Could you check a few things on this drawing? It's one solid part, dimensions in mm from its lowest x, y, z. A direction names the side the tool comes from. Coordinates: 2 decimals unless noted, no trailing zeros. Write each loop counter-clockwise with the first axis right and the second up, starting at its lowest first coordinate (ties: lowest second). Pieces come first, ordered by that corner, then holes. Notation, with made-up numbers: (69, 82.25) - (90, 82.25) arc R29 cw to (90, 119.25) - close; hole circle Ø6 at (-36.5, 69). An arc over 180 degrees is marked (long way). Answer as a JSON object with one key per item and string values. Group by question number.
1) On a 3-axis mill with a long thin cutter (end or side, diameter ignored), from which of +Z, -Z, +X, -X, +Y, -Y can I reach the whole of each face in a straight line? I mean the marked faces 1, 2 and 3. Say none if no direction works.
2) If we section it at B-B (z = 24.5): Write out the boundary of the cut face in (x, y) (1 decimal), plus the area to 3 significant figures.
3) Will these pins go through, and if not, where does the flat tip stop? pin 1 Ø1 at (y, z) = (16, 169) entering from +X; pin 2 Ø1.5 at (y, z) = (13.5, 65) entering from -X; pin 3 Ø1.2 at (y, z) = (2, 23.5) entering from +X.
4) If we section it at C-C (x = 253): Write out the boundary of the cut face in (y, z), plus the area to 3 significant figures.
5) Please list where these lines run through material, in increasing order: line 1 along Z through (x, y) = (272, 17.5); line 2 along Y through (x, z) = (126.5, 80); line 3 along Z through (x, y) = (118, 14.75) (1 decimal).
6) If we section it at D-D (z = 106.5): Write out the boundary of the cut face in (x, y), plus the area to 3 significant figures.
7) If we section it at A-A (y = 23): Write out the boundary of the cut face in (x, z) (1 decimal), plus the area to 3 significant figures.
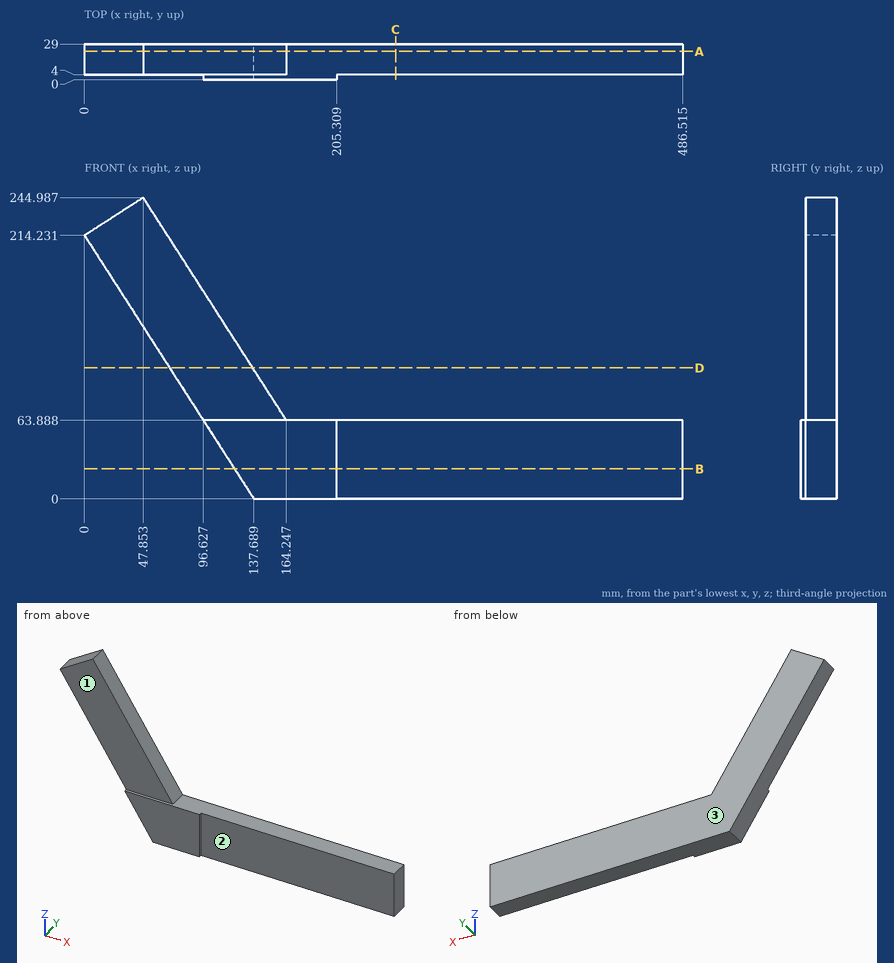
Here are the results:
{
 "1": {"face 1": "+Z, +X, -X, -Y", "face 2": "+Z, -Z, +X, -Y", "face 3": "+Z, -Z, +X, -X, +Y"},
 "2": {"outline": "(121.9, 0) - (205.3, 0) - (205.3, 4) - (486.5, 4) - (486.5, 29) - (121.9, 29) - close", "area": "9,450 mm²"},
 "3": {"pin 1": "stops at x = 97.01", "pin 2": "stops at x = 95.43", "pin 3": "stops at x = 205.31"},
 "4": {"outline": "(4, 0) - (29, 0) - (29, 63.89) - (4, 63.89) - close", "area": "1,600 mm²"},
 "5": {"line 1": "z = 0 to 63.89", "line 2": "y = 4 to 29", "line 3": "z = 30.6 to 135.8"},
 "6": {"outline": "(69.24, 4) - (136.86, 4) - (136.86, 29) - (69.24, 29) - close", "area": "1,690 mm²"},
 "7": {"outline": "(0, 214.2) - (137.7, 0) - (486.5, 0) - (486.5, 63.9) - (164.2, 63.9) - (47.9, 245) - close", "area": "34,800 mm²"}
}
